from build123d import *

# Parameters (mm, degrees)
BLANKSKE_W              = 43
BLANKSKE_H              = 16.5
BLANK_DEPTH             = 6
TOOTHCUTSIM_DEPTH       = 47.446205442
TEETHCUTS_COUNT         = 10
TEETHCUTS_PITCH         = 4.712388975
ESQUISSE1_R             = 1.5
ENL_V_MAT_EXTRU_1_DEPTH = 6


with BuildPart() as part:
    # BlankSke → Blank (new body)
    with BuildSketch(Plane.XY):
        with Locations((21.5, 8.25)):
            Rectangle(BLANKSKE_W, BLANKSKE_H)
    extrude(amount=-BLANK_DEPTH)

    # TooCutSkeSim → ToothCutSim (cut, through all)
    with BuildSketch(Plane.XY):
        Polygon((0.654653055, 13.125), (-0.654653055, 13.125), (-1.892297439, 16.5254), (1.892297439, 16.5254), align=None)
    toothcutsim = extrude(amount=-TOOTHCUTSIM_DEPTH, mode=Mode.SUBTRACT)

    # TeethCuts: ToothCutSim ×10
    with Locations(*[(i * TEETHCUTS_PITCH, 0, 0) for i in range(1, TEETHCUTS_COUNT)]):
        add(toothcutsim, mode=Mode.SUBTRACT)

    # Esquisse1 → Enlèv. mat.-Extru.1 (cut)
    with BuildSketch(Plane.XY):
        with Locations((5, 6)):
            Circle(ESQUISSE1_R)
        with Locations((19, 6)):
            Circle(ESQUISSE1_R)
    extrude(amount=-ENL_V_MAT_EXTRU_1_DEPTH, mode=Mode.SUBTRACT)


solid = part.part
Build history of the part. All positions in model axes, mm. A direction names the side the tool comes from. Give positions to 0.01 mm unless a question says otherwise; leave off trailing zeros. Order: outer loops, then holes, each group sorted by start corner. A loop starts at its lowest first (then second) coordinate and runs counter-clockwise, first axis right, second up. Notation, with made-up numbers: M 15,59.25 L 48,59.25 A9 cw 48,71.25 Z; hole C 40,89.5 d7. An arc over 180 degrees is marked long. Put each result on its own line as item: value.
Item 1: Cut at B-B on y = 6. Write the cut outline in (x, z).
Results are:
outline: M 0,-6 L 3.5,-6 L 3.5,0 L 0,0 Z; M 6.5,-6 L 17.5,-6 L 17.5,0 L 6.5,0 Z; M 20.5,-6 L 43,-6 L 43,0 L 20.5,0 Z
Item 2: Pull direction Y, two halves, no side cores. Call faces 1 (the face through (6.386, 5.425, -2.958)), 2 (the face through (24, 13.125, -3)), 3 (the face through (21, 0, -3)): +Y half, -Y half, draft (parallel to the pull), parting line (faces both ways), or undercut.
Results are:
face 1: undercut
face 2: +Y half
face 3: -Y half
Item 3: Cut at A-A on x = 19. Write the cut outline in (y, z) (3 decimals), then the cut area to 4 significant figures.
Results are:
outline: M 0,-6 L 4.5,-6 L 4.5,0 L 0,0 Z; M 7.5,-6 L 13.125,-6 L 13.125,0 L 7.5,0 Z
area: 60.75 mm2
Item 4: Wall check: probe 1 along Y at (x, z) = (5, -2.1) (3 decimals); probe 2 along Y at (x, z) = (24, -0.6) (3 decimals); probe 3 along X at (y, z) = (7.25, -4.65). Give the ranges that are in metal, low to high.
Results are:
probe 1: 0 to 4.5, 7.5 to 13.125
probe 2: 0 to 13.125
probe 3: 0 to 4.17, 5.83 to 18.17, 19.83 to 43
Item 5: Cut at C-C on z = -0.55. Count the separate pieces of the cut face and the enclosed holes in it, then the cut area to 3 significant figures.
Results are:
separate pieces: 1
enclosed holes: 2
area: 616 mm2
Item 6: Drop flat-ended pins along their axis: pin 1 Ø1 at (y, z) = (15, -1.5) entering from +X; pin 2 Ø1 at (x, z) = (33, -4.5) entering from +Y (3 decimals). Give the stop position or say it passes through.
Results are:
pin 1: x = 41.26
pin 2: y = 13.125
Item 7: Which spindle directions (+Z, -Z, +X, -X, +Y, -Y) get a long thin tool onto all of the face, cutting with end or side? Do faces 4 (the face through (30.6, 16.5, -3)), 5 (the face through (38, 13.125, -3)). Say none if no direction does.
Results are:
face 4: +Z, -Z, +X, -X, +Y
face 5: +Z, -Z, +Y
